```python
from build123d import *

# Parameters (mm, degrees)
SKETCH1_R           = 7.5
BOSS_EXTRUDE1_DEPTH = 1200
SKETCH2_OUTSIDE_W   = 257.038
SKETCH2_OUTSIDE_H   = 257.038
SKETCH2_OUTSIDE_R   = 5
CUT_EXTRUDE1_DEPTH  = 25
SKETCH3_OUTSIDE_W   = 257.038
SKETCH3_OUTSIDE_H   = 257.038
SKETCH3_OUTSIDE_R   = 5
CUT_EXTRUDE2_DEPTH  = 25


with BuildPart() as part:
    # Sketch1 → Boss-Extrude1 (new body)
    with BuildSketch(Plane(origin=(0, 0, 0), x_dir=(1, 0, 0), z_dir=(0, 1, 0))):
        Circle(SKETCH1_R)
    extrude(amount=BOSS_EXTRUDE1_DEPTH)

    # Sketch2 outside → Cut-Extrude1 (cut)
    with BuildSketch(Plane(origin=(0, 1200, 0), x_dir=(1, 0, 0), z_dir=(0, 1, 0))):
        Rectangle(SKETCH2_OUTSIDE_W, SKETCH2_OUTSIDE_H)
        Circle(SKETCH2_OUTSIDE_R, mode=Mode.SUBTRACT)
    extrude(amount=-CUT_EXTRUDE1_DEPTH, mode=Mode.SUBTRACT)

    # Sketch3 outside → Cut-Extrude2 (cut)
    with BuildSketch(Plane.XZ):
        Rectangle(SKETCH3_OUTSIDE_W, SKETCH3_OUTSIDE_H)
        Circle(SKETCH3_OUTSIDE_R, mode=Mode.SUBTRACT)
    extrude(amount=-CUT_EXTRUDE2_DEPTH, mode=Mode.SUBTRACT)


solid = part.part
```
Could you check a few things on this model? Use its own coordinates, in mm. Coordinates: 2 decimals unless noted, no trailing zeros. Order: outer loops, then holes, each group sorted by start corner. A loop starts at its lowest first (then second) coordinate and runs counter-clockwise, first axis right, second up. Notation, with made-up numbers: M 78,61.25 L 113,61.25 A17 cw 113,78.25 Z; hole C 65.25,47.25 d8. An arc over 180 degrees is marked long. Use one line per item in the form item = value. Start each with the question number.
1. For pin 1 (1.5 mm diameter, centred on y = 231.5, z = -3.5, fed in from -X); pin 2 (3 mm diameter, centred on y = 161, z = 4.5, fed in from +X); pin 3 (6 mm diameter, centred on y = 402, z = 4.5, fed in from -X), each with a flat end and sliding along its axis, tell me the tip position at first contact or that it passes through.
2. Suppose I cut it at C-C on y = 414.5. Write out the boundary of the cut face in (x, z), then the cut area to 3 significant figures.
3. Suppose I cut it at B-B on x = 2. Write out the boundary of the cut face in (y, z).
4. Please list where these lines run through material, in increasing order: line 1 (X direction, y = 959.5, z = 1.5); line 2 (Z direction, x = -1, y = 837.5); line 3 (Y direction, x = -1.5, z = -5.75).
5. Suppose I cut it at A-A on z = 2.75. Write out the boundary of the cut face in (x, y), then the cut area to 3 significant figures.
Geometry says:
q1.pin_1 = -6.98
q1.pin_2 = 6.87
q1.pin_3 = -7.35
q2.outline = C 0,0 d15
q2.area = 177 mm^2
q3.outline = M 0,-4.58 L 25,-4.58 L 25,-7.23 L 1175,-7.23 L 1175,-4.58 L 1200,-4.58 L 1200,4.58 L 1175,4.58 L 1175,7.23 L 25,7.23 L 25,4.58 L 0,4.58 Z
q4.line_1 = -7.35 to 7.35
q4.line_2 = -7.43 to 7.43
q4.line_3 = 25 to 1175
q5.outline = M -6.98,25 L -4.18,25 L -4.18,0 L 4.18,0 L 4.18,25 L 6.98,25 L 6.98,1175 L 4.18,1175 L 4.18,1200 L -4.18,1200 L -4.18,1175 L -6.98,1175 Z
q5.area = 16,500 mm^2
